Design review of the part built by this model. Coordinates are the model's own, in mm. A direction names the side the tool comes from. Coordinates: 2 decimals unless noted, no trailing zeros. Write each loop counter-clockwise with the first axis right and the second up, starting at its lowest first coordinate (ties: lowest second). Pieces come first, ordered by that corner, then holes. Notation, with made-up numbers: M -33,68.5 L -13,68.5 A36 ccw -13,104.5 Z; hole C 55,-8.75 d3. An arc over 180 degrees is marked long. Write item = value, one per line.
```python
from build123d import *

# Parameters (mm, degrees)
SKETCH2_W           = 300
SKETCH2_H           = 300
BOSS_EXTRUDE1_DEPTH = 150
SKETCH4_R           = 20
CUT_EXTRUDE1_DEPTH  = 368.423461417
SKETCH8_R           = 50
BOSS_EXTRUDE3_DEPTH = 40
SKETCH10_R          = 50
BOSS_EXTRUDE4_DEPTH = 50
FILLET1_R           = 49


with BuildPart() as part:
    # Sketch2 → Boss-Extrude1 (new body)
    with BuildSketch(Plane(origin=(0, 0, 0), x_dir=(1, 0, 0), z_dir=(0, 1, 0))):
        Rectangle(SKETCH2_W, SKETCH2_H)
    extrude(amount=BOSS_EXTRUDE1_DEPTH)

    # Sketch4 → Cut-Extrude1 (cut, through all)
    with BuildSketch(Plane.XY.offset(150)):
        with Locations((-50, 40)):
            Circle(SKETCH4_R)
    extrude(amount=-CUT_EXTRUDE1_DEPTH, mode=Mode.SUBTRACT)

    # Sketch8 → Boss-Extrude3 (add)
    with BuildSketch(Plane(origin=(0, 150, 0), x_dir=(1, 0, 0), z_dir=(0, 1, 0))):
        with Locations(Location((0, 0, 0), (0, 0, 270))):
            Circle(SKETCH8_R)
    extrude(amount=BOSS_EXTRUDE3_DEPTH)

    # Sketch10 → Boss-Extrude4 (add)
    with BuildSketch(Plane(origin=(0, 0, 0), x_dir=(-1, 0, 0), z_dir=(0, -1, 0))):
        with Locations(Location((-90, 0, 0), (0, 0, 270))):
            Circle(SKETCH10_R)
    extrude(amount=BOSS_EXTRUDE4_DEPTH)

    # Fillet1
    fillet1_edges = [part.edges().sort_by_distance(p)[0] for p in [
        (90, -50, -50),
    ]]
    fillet(fillet1_edges, radius=FILLET1_R)


solid = part.part
```
Q1. For P1, Ø5, axis at x = 96, z = 43, coming from the -Y side; P2, Ø1, axis at x = 115.5, z = -11, coming from the -Y side; P3, Ø1.5, axis at x = -38, z = 24, coming from the -Y side, all flat-tipped, find the tip position at first contact; note any pin that passes through.
Check result:
P1 = -29.42
P2 = -42.36
P3 = 0
Q2. Consider section B-B, the plane z = 107. State the section outline as (x, y) points, and give its area (3 significant figures).
Check result:
outline = M -150,0 L 150,0 L 150,150 L -150,150 Z; hole C -50,40 d40
area = 43,700 mm²
Q3. Consider section A-A, the plane y = 40. State the section outline as (x, z) points.
Check result:
outline = M -150,-150 L -70,-150 L -70,150 L -150,150 Z; M -30,-150 L 150,-150 L 150,150 L -30,150 Z
Q4. Wall thickness on line 1 (Y direction, x = -50, z = -56); line 2 (Y direction, x = 30, z = 51.5); line 3 (Z direction, x = 98.5, y = -26): over which ranges is each line inside the solid? List them lowest first.
Check result:
line_1 = 0 to 20, 60 to 150
line_2 = 0 to 150
line_3 = -42.3 to 42.3
Q5. Machinability: for faces 4 (the flat face through (150, 74, 2)), 5 (the cylindrical face through (15.02, 169.72, 47.69)), 6 (the cylindrical face through (138.81, -0.49, -10.84)), which of the approach directions +Z, -Z, +X, -X, +Y, -Y give a long, thin tool a straight path to every point of the face, cutting with its end or side? Answer none if there is none.
Check result:
face_4 = +Z, -Z, +X, +Y, -Y
face_5 = +Y
face_6 = -Y
Q6. Consider section C-C, the plane x = 0. State the section outline as (y, z) points, and give its area (3 significant figures).
Check result:
outline = M 0,-150 L 150,-150 L 150,-50 L 190,-50 L 190,50 L 150,50 L 150,150 L 0,150 Z
area = 49,000 mm²
Q7. Consider section D-D, the plane y = 156. State the section outline as (x, z) points, and give its area (3 significant figures).
Check result:
outline = C 0,0 d100
area = 7,850 mm²
Q8. The part is to be moulded in two halves that separate along Y. For faces 1 (the flat face through (-2, 74, -150)), 2 (the flat face through (1, 190, -1)), 3 (the cylindrical face through (-30.924, 46.007, 2.1)), say which applies: +Y half, -Y half, draft (parallel to the pull), parting line (faces both ways), or undercut.
Check result:
face_1 = draft
face_2 = +Y half
face_3 = undercut
